Here's how the part is built. I have some questions about the finished solid (model axes, mm). A direction names the side the tool comes from. Coordinates: 2 decimals unless noted, no trailing zeros. Order: outer loops, then holes, each group sorted by start corner. A loop starts at its lowest first (then second) coordinate and runs counter-clockwise, first axis right, second up. Notation, with made-up numbers: (39, -24.75) - (81, -24.75) arc R10 cw to (81, -7.75) - close; hole circle Ø2 at (25.5, 71). An arc over 180 degrees is marked (long way). Answer as CSV lines item,"result". Start each with the question number.
Q1. Suppose I cut it at C-C (z = 4). Please give me the cut outline in (x, y) (3 decimals).
Q2. Suppose I cut it at D-D (z = 10.5). Please give me the cut outline in (x, y).
Q3. For pin 1 Ø2 at (y, z) = (-5.5, 12) entering from +X; pin 2 Ø3 at (x, y) = (6.5, 6.5) entering from +Z; pin 3 Ø3 at (x, y) = (6.12, 5.3) entering from -Z, each with a flat end and sliding along its axis, tell me the tip position at first contact or that it passes through.
Q4. I need wall thicknesses on line 1 (Z direction, x = 5.25, y = 1.5); line 2 (Z direction, x = 5, y = -11.5); line 3 (Y direction, x = 1, z = 32.5). Which ranges of each line are inside material? Lowest first, please.
Q5. For faces 4 (the face through (2, 3, 25)), 5 (the face through (4.87, 6.45, 2.68)), 6 (the face through (0, 0, 0)), which set-ups out of +Z, -Z, +X, -X, +Y, -Y let a thin tool reach every point of the face, with its end or its side?
Q6. Suppose I cut it at A-A (x = 0). Please give me the cut outline in (y, z), then the cut area to 3 significant figures.
Q7. Thinking about a two-plate mould opening in Y: for faces 1 (the face through (-6.22, 10.324, 20.5)), 2 (the face through (-8.771, 8.043, 22.782)), 3 (the face through (5.85, -5.42, 5.84)), which applies, released by +Y, released by -Y, zero draft, split by the parting line, or undercut?
from build123d import *

# Parameters (mm, degrees)
SKETCH1_R                                       = 13.85
BOSS_EXTRUDE1_DEPTH                             = 25
SKETCH2_OUTSIDE_W                               = 38.994
SKETCH2_OUTSIDE_H                               = 38.994
SKETCH2_OUTSIDE_R                               = 11.9
CUT_EXTRUDE3_DEPTH                              = 4.5
SKETCH6_OUTSIDE_W                               = 38.994
SKETCH6_OUTSIDE_H                               = 38.994
SKETCH6_OUTSIDE_R                               = 12.25
CUT_EXTRUDE5_DEPTH                              = 4.5
SKETCH7_R                                       = 3.45
BOSS_EXTRUDE2_DEPTH                             = 14
CSK_FOR_M3_OVAL_HEAD_MACHINE_SCREW2_D           = 3.4
CSK_FOR_M3_OVAL_HEAD_MACHINE_SCREW2_DEPTH       = 5
CSK_FOR_M3_OVAL_HEAD_MACHINE_SCREW2_CSINK_D     = 4
CSK_FOR_M3_OVAL_HEAD_MACHINE_SCREW2_CSINK_ANGLE = 90
CSK_FOR_M3_OVAL_HEAD_MACHINE_SCREW2_TIP         = 1.021463052


with BuildPart() as part:
    # Sketch1 → Boss-Extrude1 (new body)
    with BuildSketch(Plane.XY):
        Circle(SKETCH1_R)
    extrude(amount=BOSS_EXTRUDE1_DEPTH)

    # Sketch2 outside → Cut-Extrude3 (cut)
    with BuildSketch(Plane.XY.offset(25)):
        Rectangle(SKETCH2_OUTSIDE_W, SKETCH2_OUTSIDE_H)
        Circle(SKETCH2_OUTSIDE_R, mode=Mode.SUBTRACT)
    extrude(amount=-CUT_EXTRUDE3_DEPTH, mode=Mode.SUBTRACT)

    # Sketch6 outside → Cut-Extrude5 (cut)
    with BuildSketch(Plane(origin=(0, 0, 0), x_dir=(-1, 0, 0), z_dir=(0, 0, -1))):
        Rectangle(SKETCH6_OUTSIDE_W, SKETCH6_OUTSIDE_H)
        Circle(SKETCH6_OUTSIDE_R, mode=Mode.SUBTRACT)
    extrude(amount=-CUT_EXTRUDE5_DEPTH, mode=Mode.SUBTRACT)

    # Sketch7 → Boss-Extrude2 (add)
    with BuildSketch(Plane.XY.offset(25)):
        Circle(SKETCH7_R)
    extrude(amount=BOSS_EXTRUDE2_DEPTH)

    # CSK for M3 Oval Head Machine Screw2
    with Locations(Plane(origin=(0, 0, 0), x_dir=(-1, 0, 0), z_dir=(0, 0, -1))):
        with Locations((-6.125, 5.304405598), (6.125, 5.304405598), (6.125, -5.304405598), (-6.125, -5.304405598)):
            CounterSinkHole(CSK_FOR_M3_OVAL_HEAD_MACHINE_SCREW2_D / 2, CSK_FOR_M3_OVAL_HEAD_MACHINE_SCREW2_CSINK_D / 2, depth=CSK_FOR_M3_OVAL_HEAD_MACHINE_SCREW2_DEPTH, counter_sink_angle=CSK_FOR_M3_OVAL_HEAD_MACHINE_SCREW2_CSINK_ANGLE)
            with Locations((0, 0, -(CSK_FOR_M3_OVAL_HEAD_MACHINE_SCREW2_DEPTH + CSK_FOR_M3_OVAL_HEAD_MACHINE_SCREW2_TIP / 2))):  # 118° drill point
                Cone(0, CSK_FOR_M3_OVAL_HEAD_MACHINE_SCREW2_D / 2, CSK_FOR_M3_OVAL_HEAD_MACHINE_SCREW2_TIP, mode=Mode.SUBTRACT)


solid = part.part
Here are the results:
1,outline,"circle Ø24.5 at (0, 0); hole circle Ø3.4 at (-6.125, -5.304); hole circle Ø3.4 at (-6.125, 5.304); hole circle Ø3.4 at (6.125, -5.304); hole circle Ø3.4 at (6.125, 5.304)"
2,outline,"circle Ø27.7 at (0, 0)"
3,pin 1,"stops at x = 13.1"
3,pin 2,"stops at z = 25"
3,pin 3,"stops at z = 5.12"
4,line 1,"z = 0 to 25"
4,line 2,"z = 4.5 to 20.5"
4,line 3,"y = -3.3 to 3.3"
5,face 4,"+Z"
5,face 5,"-Z"
5,face 6,"-Z, +X, -X, +Y, -Y"
6,outline,"(-13.85, 4.5) - (-12.25, 4.5) - (-12.25, 0) - (12.25, 0) - (12.25, 4.5) - (13.85, 4.5) - (13.85, 20.5) - (11.9, 20.5) - (11.9, 25) - (3.45, 25) - (3.45, 39) - (-3.45, 39) - (-3.45, 25) - (-11.9, 25) - (-11.9, 20.5) - (-13.85, 20.5) - close"
6,area,"757 mm²"
7,face 1,"zero draft"
7,face 2,"split by the parting line"
7,face 3,"undercut"
